```python
from build123d import *

# Parameters (mm, degrees)
F2_R      = 2
F3_DEPTH  = 3
F4_W      = 3
F4_H      = 35
F4_H_2    = 3
F4_W_2    = 41
F5_DEPTH  = 114
F6_R      = 2
F7_DEPTH  = 3
F8_W      = 110
F8_H      = 20
F9_DEPTH  = 3
F10_W     = 48
F10_H     = 27
F11_DEPTH = 3
F12_R     = 5.2787577195
F13_DEPTH = 3


with BuildPart() as f3:
    # F2 (on Right) → F3 (new body)
    with BuildSketch(Plane.YZ):
        with BuildLine():
            ThreePointArc((22.5, 35), (21.0355339059, 38.5355339059), (17.5, 40))
            Line((17.5, 40), (-19.5, 40))
            ThreePointArc((-19.5, 40), (-23.0355339059, 38.5355339059), (-24.5, 35))
            Line((-24.5, 35), (-24.5, -38))
            Line((-24.5, -38), (22.5, -38))
            Line((22.5, -38), (22.5, 35))
        make_face()
        with Locations((-12.5, 34)):
            Circle(F2_R, mode=Mode.SUBTRACT)
        with Locations((10.5, 34)):
            Circle(F2_R, mode=Mode.SUBTRACT)
    extrude(amount=F3_DEPTH)

    # F4 (on Right) → F5 (join)
    with BuildSketch(Plane.YZ):
        with Locations((-23, -17.5)):
            Rectangle(F4_W, F4_H)
        with Locations((21, -36.5)):
            Rectangle(F4_W, F4_H_2)
        with Locations((21, -17.5)):
            Rectangle(F4_W, F4_H)
        with Locations((-1, -36.5)):
            Rectangle(F4_W_2, F4_H_2)
        with Locations((-23, -36.5)):
            Rectangle(F4_W, F4_H_2)
    extrude(amount=-F5_DEPTH)

    # F6 (on face) → F7 (join)
    with BuildSketch(Plane(origin=(-114, 0, 0), x_dir=(0, -1, 0), z_dir=(-1, 0, 0))):
        with BuildLine():
            ThreePointArc((24.5, 35), (23.0355339059, 38.5355339059), (19.5, 40))
            Line((19.5, 40), (-17.5, 40))
            ThreePointArc((-17.5, 40), (-21.0355339059, 38.5355339059), (-22.5, 35))
            Line((-22.5, 35), (-22.5, -38))
            Line((-22.5, -38), (24.5, -38))
            Line((24.5, -38), (24.5, 35))
        make_face()
        with Locations((-10.5, 34)):
            Circle(F6_R, mode=Mode.SUBTRACT)
    extrude(amount=F7_DEPTH)

    # F8 (on face) → F9 (join)
    with BuildSketch(Plane.XZ.offset(24.5)):
        with Locations((-57, 10)):
            Rectangle(F8_W, F8_H)
    extrude(amount=-F9_DEPTH)

    # F10 (on face) → F11 (cut, through all)
    with BuildSketch(Plane.XZ.offset(24.5)):
        with Locations((-28.5, -19)):
            Rectangle(F10_W, F10_H)
    extrude(amount=-F11_DEPTH, mode=Mode.SUBTRACT)

    # F12 (on face) → F13 (cut, through all)
    with BuildSketch(Plane(origin=(0, 0, -38), x_dir=(1, 0, 0), z_dir=(0, 0, -1))):
        with Locations((-39.4231006503, -5.3282435983)):
            Circle(F12_R)
    extrude(amount=-F13_DEPTH, mode=Mode.SUBTRACT)


solid = f3.part
```
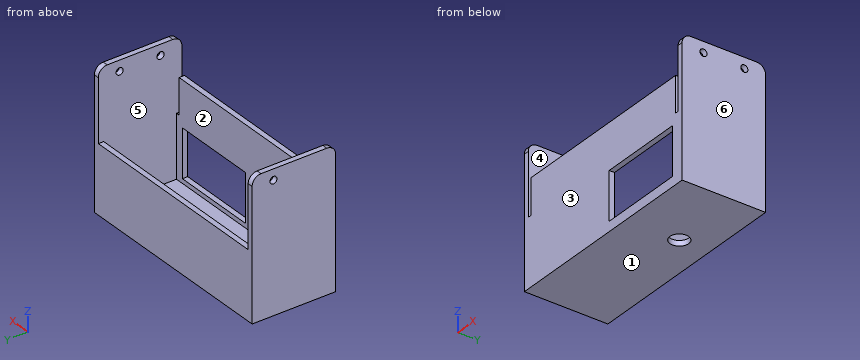
Part model, mm, in its own coordinate system. Face numbers are marked on the shaded views. A direction names the side the tool comes from. Give positions to 0.01 mm unless a question says otherwise; leave off trailing zeros. Loops run counter-clockwise (first coordinate to the right, second up) from the corner with the lowest first, then second, coordinate; pieces in that order, holes last. Notation, with made-up numbers: M -32,-14.5 L 6,-14.5 A11 ccw 6,5.5 Z; hole C 35,49.5 d8. An arc over 180 degrees is marked long. Return JSON: item names as keys, results as strings.
1) Flat gauge pins, fed straight in: pin 1 Ø2 at (x, y) = (-72.5, 0) entering from +Z; pin 2 Ø0.9 at (x, y) = (-26, -23) entering from +Z; pin 3 Ø2.5 at (x, y) = (-35.5, 21) entering from +Z; pin 4 Ø3.5 at (y, z) = (10.5, 34) entering from -X. Where does each tip first touch, or does it go through?
Calculated:
{"pin 1": "stops at z = -35", "pin 2": "stops at z = 20", "pin 3": "stops at z = 0", "pin 4": "passes through"}
2) Drill centre lines: line 1 (Z direction, x = -115.8, y = 10.5); line 2 (X direction, y = -8.5, z = -17); line 3 (Y direction, x = -67, z = -21). Where is each one in solid material? Low to high.
Calculated:
{"line 1": "z = -38 to 32, 36 to 40", "line 2": "x = -117 to -114, 0 to 3", "line 3": "y = -24.5 to -21.5, 19.5 to 22.5"}
3) Saw through at A-A, the plane z = 12. List the corners of the cut face in (x, y), then the cut area to 3 significant figures.
Calculated:
{"outline": "M -117,-24.5 L -114,-24.5 L -114,22.5 L -117,22.5 Z; M -112,-24.5 L -2,-24.5 L -2,-21.5 L -112,-21.5 Z; M 0,-24.5 L 3,-24.5 L 3,22.5 L 0,22.5 Z", "area": "612 mm2"}
4) Pull direction Y, two halves, no side cores. Call the marked faces 1, 2, 3 and 4: released by +Y, released by -Y, zero draft, split by the parting line, or undercut.
Calculated:
{"face 1": "zero draft", "face 2": "undercut", "face 3": "released by -Y", "face 4": "undercut"}
5) Saw through at C-C, the plane y = -12.5. List the corners of the cut face in (x, z), then the cut area to 3 significant figures.
Calculated:
{"outline": "M -117,-38 L 3,-38 L 3,32 L 0,32 L 0,-35 L -114,-35 L -114,40 L -117,40 Z; M 0,36 L 3,36 L 3,40 L 0,40 Z", "area": "798 mm2"}
6) Saw through at D-D, the plane z = 29. List the corners of the cut face in (x, y), then the cut area to 3 significant figures.
Calculated:
{"outline": "M -117,-24.5 L -114,-24.5 L -114,22.5 L -117,22.5 Z; M 0,-24.5 L 3,-24.5 L 3,22.5 L 0,22.5 Z", "area": "282 mm2"}
7) Saw through at B-B, the plane x = -8.5. List the corners of the cut face in (y, z), then the cut area to 3 significant figures.
Calculated:
{"outline": "M -24.5,-38 L 22.5,-38 L 22.5,0 L 19.5,0 L 19.5,-35 L -21.5,-35 L -21.5,-32.5 L -24.5,-32.5 Z; M -24.5,-5.5 L -21.5,-5.5 L -21.5,20 L -24.5,20 Z", "area": "330 mm2"}
8) 3-axis set-ups, long thin cutter, end or side, ignore diameter. For the marked faces 5 and 6: which of +Z, -Z, +X, -X, +Y, -Y reach the whole face in a straight line?
Calculated:
{"face 5": "+Z", "face 6": "+Z, -Z, +X, +Y, -Y"}
